```python
from build123d import *

# Parameters (mm, degrees)
F0_W      = 69.85
F0_H      = 44.45
F1_DEPTH  = 3.175
F2_W      = 69.85
F2_H      = 44.45
F2_W_2    = 63.5
F2_H_2    = 38.1
F3_DEPTH  = 25.273
F5_DEPTH  = 38.1
F6_R      = 0.79375
F7_DEPTH  = 1.5875
F8_W      = 69.85
F8_H      = 44.45
F9_DEPTH  = 6.35
F10_W     = 63.5
F10_H     = 3.175
F11_DEPTH = 3.175
F12_W     = 63.5
F12_H     = 3.175
F13_DEPTH = 3.175
F14_W     = 31.75
F14_H     = 3.175
F15_DEPTH = 3.175
F16_W     = 69.85
F16_H     = 3.175
F17_DEPTH = 6.223
F18_W     = 69.85
F18_H     = 3.048
F19_DEPTH = 3.048
F20_W     = 69.85
F20_H     = 3.048
F21_DEPTH = 3.048
F22_W     = 3.302
F22_H     = 6.223
F23_DEPTH = 38.1


with BuildPart() as f1:
    # F0 (on Top) → F1 (new body)
    with BuildSketch(Plane.XY):
        with Locations((34.925, -22.225)):
            Rectangle(F0_W, F0_H)
    extrude(amount=F1_DEPTH)

    # F2 (on face) → F3 (join)
    with BuildSketch(Plane.XY.offset(3.175)):
        with Locations((34.925, -22.225)):
            Rectangle(F2_W, F2_H)
        with Locations((34.925, -22.225)):
            Rectangle(F2_W_2, F2_H_2, mode=Mode.SUBTRACT)
    extrude(amount=F3_DEPTH)

    # F4 (on face) → F5 (join, through all)
    with BuildSketch(Plane.XZ.offset(3.175)):
        Polygon((34.925, 19.2405), (34.925, 20.828), (24.765, 20.828), (18.9080913895, 28.448), (16.9058381181, 28.448), (23.9829360225, 19.2405), (33.274, 19.2405), align=None)
        Polygon((45.085, 20.828), (34.925, 20.828), (34.925, 19.2405), (45.8670639775, 19.2405), (52.9441618819, 28.448), (50.9419086105, 28.448), align=None)
    extrude(amount=F5_DEPTH)

    # F6 (on face) → F7 (cut, through all)
    with BuildSketch(Plane.XY.offset(20.828)):
        with Locations((27.3135136813, -6.1057861894)):
            Circle(F6_R)
        with Locations((29.8535136813, -6.1057861894)):
            Circle(F6_R)
        with Locations((32.3935136813, -6.1057861894)):
            Circle(F6_R)
        with Locations((27.305, -9.7028)):
            Circle(F6_R)
        with Locations((29.845, -9.7028)):
            Circle(F6_R)
        with Locations((32.385, -9.7028)):
            Circle(F6_R)
        with Locations((27.2964863187, -13.2998138106)):
            Circle(F6_R)
        with Locations((29.8364863187, -13.2998138106)):
            Circle(F6_R)
        with Locations((32.3764863187, -13.2998138106)):
            Circle(F6_R)
        with Locations((27.2879726374, -16.8968276211)):
            Circle(F6_R)
        with Locations((29.8279726374, -16.8968276211)):
            Circle(F6_R)
        with Locations((32.3679726374, -16.8968276211)):
            Circle(F6_R)
        with Locations((27.2794589561, -20.4938414317)):
            Circle(F6_R)
        with Locations((29.8194589561, -20.4938414317)):
            Circle(F6_R)
        with Locations((32.3594589561, -20.4938414317)):
            Circle(F6_R)
        with Locations((42.5364863187, -6.1057861894)):
            Circle(F6_R)
        with Locations((39.9964863187, -6.1057861894)):
            Circle(F6_R)
        with Locations((37.4564863187, -6.1057861894)):
            Circle(F6_R)
        with Locations((37.465, -9.7028)):
            Circle(F6_R)
        with Locations((40.005, -9.7028)):
            Circle(F6_R)
        with Locations((42.545, -9.7028)):
            Circle(F6_R)
        with Locations((42.5535136813, -13.2998138106)):
            Circle(F6_R)
        with Locations((40.0135136813, -13.2998138106)):
            Circle(F6_R)
        with Locations((37.4735136813, -13.2998138106)):
            Circle(F6_R)
        with Locations((42.5620273626, -16.8968276211)):
            Circle(F6_R)
        with Locations((40.0220273626, -16.8968276211)):
            Circle(F6_R)
        with Locations((37.4820273626, -16.8968276211)):
            Circle(F6_R)
        with Locations((42.5705410439, -20.4938414317)):
            Circle(F6_R)
        with Locations((40.0305410439, -20.4938414317)):
            Circle(F6_R)
        with Locations((37.4905410439, -20.4938414317)):
            Circle(F6_R)
        with Locations((27.2794589561, -23.9561585683)):
            Circle(F6_R)
        with Locations((29.8194589561, -23.9561585683)):
            Circle(F6_R)
        with Locations((32.3594589561, -23.9561585683)):
            Circle(F6_R)
        with Locations((27.2879726374, -27.5531723789)):
            Circle(F6_R)
        with Locations((29.8279726374, -27.5531723789)):
            Circle(F6_R)
        with Locations((32.3679726374, -27.5531723789)):
            Circle(F6_R)
        with Locations((32.3764863187, -31.1501861894)):
            Circle(F6_R)
        with Locations((29.8364863187, -31.1501861894)):
            Circle(F6_R)
        with Locations((27.2964863187, -31.1501861894)):
            Circle(F6_R)
        with Locations((27.305, -34.7472)):
            Circle(F6_R)
        with Locations((29.845, -34.7472)):
            Circle(F6_R)
        with Locations((32.385, -34.7472)):
            Circle(F6_R)
        with Locations((32.3935136813, -38.3442138106)):
            Circle(F6_R)
        with Locations((29.8535136813, -38.3442138106)):
            Circle(F6_R)
        with Locations((27.3135136813, -38.3442138106)):
            Circle(F6_R)
        with Locations((37.4564863187, -38.3442138106)):
            Circle(F6_R)
        with Locations((39.9964863187, -38.3442138106)):
            Circle(F6_R)
        with Locations((42.5364863187, -38.3442138106)):
            Circle(F6_R)
        with Locations((37.465, -34.7472)):
            Circle(F6_R)
        with Locations((40.005, -34.7472)):
            Circle(F6_R)
        with Locations((42.545, -34.7472)):
            Circle(F6_R)
        with Locations((37.4735136813, -31.1501861894)):
            Circle(F6_R)
        with Locations((40.0135136813, -31.1501861894)):
            Circle(F6_R)
        with Locations((42.5535136813, -31.1501861894)):
            Circle(F6_R)
        with Locations((37.4820273626, -27.5531723789)):
            Circle(F6_R)
        with Locations((40.0220273626, -27.5531723789)):
            Circle(F6_R)
        with Locations((42.5620273626, -27.5531723789)):
            Circle(F6_R)
        with Locations((37.4905410439, -23.9561585683)):
            Circle(F6_R)
        with Locations((40.0305410439, -23.9561585683)):
            Circle(F6_R)
        with Locations((42.5705410439, -23.9561585683)):
            Circle(F6_R)
    extrude(amount=-F7_DEPTH, mode=Mode.SUBTRACT)

    # F8 (on face) → F9 (join)
    with BuildSketch(Plane.XY.offset(28.448)):
        with Locations((34.925, -22.225)):
            Rectangle(F8_W, F8_H)
        Polygon((18.9080913895, -41.275), (16.9058381181, -41.275), (3.175, -41.275), (3.175, -3.175), (16.9058381181, -3.175), (18.9080913895, -3.175), (50.9419086105, -3.175), (52.9441618819, -3.175), (66.675, -3.175), (66.675, -41.275), (52.9441618819, -41.275), (50.9419086105, -41.275), align=None, mode=Mode.SUBTRACT)
    extrude(amount=F9_DEPTH)

    # F10 (on face) → F11 (join)
    with BuildSketch(Plane(origin=(0, -41.275, 0), x_dir=(-1, 0, 0), z_dir=(0, 1, 0))):
        with Locations((-34.925, 33.2105)):
            Rectangle(F10_W, F10_H)
    extrude(amount=F11_DEPTH)

    # F12 (on face) → F13 (join)
    with BuildSketch(Plane.XZ.offset(3.175)):
        with Locations((34.925, 33.2105)):
            Rectangle(F12_W, F12_H)
    extrude(amount=F13_DEPTH)

    # F14 (on face) → F15 (cut, through all)
    with BuildSketch(Plane.YZ.offset(69.85)):
        with Locations((-22.225, 33.2105)):
            Rectangle(F14_W, F14_H)
        Polygon((-6.35, 31.623), (-38.1, 31.623), (-41.275, 31.623), (-41.275, 28.448), (-3.175, 28.448), (-3.175, 31.623), align=None)
    extrude(amount=-F15_DEPTH, mode=Mode.SUBTRACT)

    # F16 (on face) → F17 (join)
    with BuildSketch(Plane(origin=(0, 0, 0), x_dir=(1, 0, 0), z_dir=(0, 0, -1))):
        with Locations((34.925, 7.9375)):
            Rectangle(F16_W, F16_H)
        with Locations((34.925, 36.5125)):
            Rectangle(F16_W, F16_H)
    extrude(amount=F17_DEPTH)

    # F18 (on face) → F19 (join)
    with BuildSketch(Plane.XZ.offset(38.1)):
        with Locations((34.925, -4.699)):
            Rectangle(F18_W, F18_H)
    extrude(amount=F19_DEPTH)

    # F20 (on face) → F21 (join)
    with BuildSketch(Plane(origin=(0, -6.35, 0), x_dir=(-1, 0, 0), z_dir=(0, 1, 0))):
        with Locations((-34.925, -4.699)):
            Rectangle(F20_W, F20_H)
    extrude(amount=F21_DEPTH)

    # F22 (on face) → F23 (cut)
    with BuildSketch(Plane.XZ.offset(41.148)):
        with Locations((1.651, -3.1115)):
            Rectangle(F22_W, F22_H)
    extrude(amount=-F23_DEPTH, mode=Mode.SUBTRACT)


solid = f1.part
```
Work out the finished part from the listing and answer in its coordinate system (mm). A direction names the side the tool comes from. Coordinates: 2 decimals unless noted, no trailing zeros. Write each loop counter-clockwise with the first axis right and the second up, starting at its lowest first coordinate (ties: lowest second). Pieces come first, ordered by that corner, then holes. Notation, with made-up numbers: (89.5, 12) - (141.5, 12) arc R16 ccw to (141.5, 19) - close; hole circle Ø2 at (65, -37). An arc over 180 degrees is marked (long way). Answer as a JSON object with one key per item and string values.
Q1. Find section C-C (z = 4). Write down the section's boundary in (x, y) (3 decimals).
Results list:
{"outline": "(0, -44.45) - (69.85, -44.45) - (69.85, 0) - (0, 0) - close; hole (3.175, -41.275) - (66.675, -41.275) - (66.675, -3.175) - (3.175, -3.175) - close"}
Q2. Which of the six approach directions +Z, -Z, +X, -X, +Y, -Y give full straight-line access (tool end or side, diameter ignored) to faces 4 (the flat face through (36, -34.925, -3)), 5 (the cylindrical face through (29.026, -20.459, 20.045)), 6 (the flat face through (37, -41.275, 17))?
Results list:
{"face 4": "-Z, +X, -X", "face 5": "+Z", "face 6": "none"}
Q3. Find section B-B (z = -1). Write down the section's boundary in (x, y) (3 decimals).
Results list:
{"outline": "(3.302, -38.1) - (69.85, -38.1) - (69.85, -34.925) - (3.302, -34.925) - close; (3.302, -9.525) - (69.85, -9.525) - (69.85, -6.35) - (3.302, -6.35) - close"}
Q4. Given pin 1 Ø1 at (x, y) = (38, -32) entering from +Z; pin 2 Ø2 at (x, y) = (32.36, -23.96) entering from -Z; pin 3 Ø3.5 at (x, z) = (45, -5) entering from +Y, each flat-ended and moving along its own axis, determine where each tip first touches the part or whether it passes through.
Results list:
{"pin 1": "stops at z = 20.83", "pin 2": "stops at z = 0", "pin 3": "stops at y = -3.3"}
Q5. Find section D-D (x = 58.5). Write down the section's boundary in (y, z) (3 decimals), plus the area to 3 significant figures.
Results list:
{"outline": "(-44.45, 0) - (-38.1, 0) - (-38.1, -3.175) - (-41.148, -3.175) - (-41.148, -6.223) - (-34.925, -6.223) - (-34.925, 0) - (-9.525, 0) - (-9.525, -6.223) - (-3.302, -6.223) - (-3.302, -3.175) - (-6.35, -3.175) - (-6.35, 0) - (0, 0) - (0, 34.798) - (-6.35, 34.798) - (-6.35, 31.623) - (-3.175, 31.623) - (-3.175, 3.175) - (-41.275, 3.175) - (-41.275, 31.623) - (-38.1, 31.623) - (-38.1, 34.798) - (-44.45, 34.798) - close", "area": "420 mm^2"}
Q6. For a pull along Y with two mould halves and no side action, classify faces 1 (the flat face through (36, -38.1, -2)), 2 (the cylindrical face through (37.31, -28.33, 20.05)), 3 (the flat face through (3.302, -37, -4)) as pulls with the +Y half, pulls with the -Y half, needs draft (parallel to the pull), parting line crosses it, or undercut.
Results list:
{"face 1": "pulls with the -Y half", "face 2": "undercut", "face 3": "needs draft"}
Q7. Consider L1, parallel to Z at x = 32.5, y = -40 (1 decimal); L2, parallel to Y at x = 52.5, z = 12 (3 decimals); L3, parallel to Y at x = 59, z = -5 (3 decimals). Determine where each line is inside the solid, lowest interval first. Write a range as from..to.
Results list:
{"L1": "z = -6.2..-3.2, 0..3.2, 19.2..20.8, 31.6..34.8", "L2": "y = -44.45..-41.275, -3.175..0", "L3": "y = -41.148..-34.925, -9.525..-3.302"}
